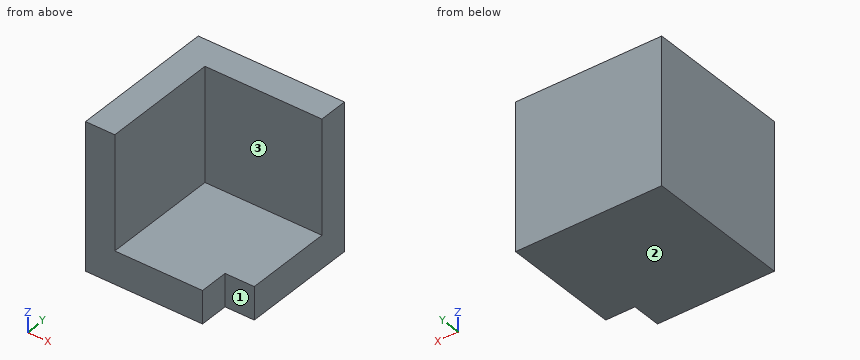
```python
from build123d import *

# Parameters (mm, degrees)
F0_W     = 63.5
F0_H     = 63.5
F1_DEPTH = 63.5
F2_W     = 50.8
F2_H     = 50.8
F3_DEPTH = 49.293023
F4_W     = 12.7
F4_H     = 12.7
F5_DEPTH = 25.4


with BuildPart() as f1:
    # F0 (on Front) → F1 (new body)
    with BuildSketch(Plane.XZ):
        with Locations((31.75, 31.75)):
            Rectangle(F0_W, F0_H)
    extrude(amount=F1_DEPTH)

    # F2 (on face) → F3 (cut)
    with BuildSketch(Plane.XY.offset(63.5)):
        with Locations((38.1, -38.1)):
            Rectangle(F2_W, F2_H)
    extrude(amount=-F3_DEPTH, mode=Mode.SUBTRACT)

    # F4 (on face) → F5 (cut)
    with BuildSketch(Plane.XY.offset(14.206977)):
        with Locations((57.15, -57.15)):
            Rectangle(F4_W, F4_H)
    extrude(amount=-F5_DEPTH, mode=Mode.SUBTRACT)


solid = f1.part
```
Here's how the part is built. I have some questions about the finished solid (model axes, mm). Face numbers are marked on the shaded views. A direction names the side the tool comes from. Round coordinates to 2 decimals unless told otherwise and drop trailing zeros. Order: outer loops, then holes, each group sorted by start corner. A loop starts at its lowest first (then second) coordinate and runs counter-clockwise, first axis right, second up. Notation, with made-up numbers: M 73.5,74.5 L 109.5,74.5 A36 ccw 109.5,108.5 Z; hole C 50.5,-35.75 d11. An arc over 180 degrees is marked long. Answer in a Markdown table with one row per item.
Item 1: Imagine slicing it at B-B, the plane x = 56.5. Write out the boundary of the cut face in (y, z).
A:
| item | result |
|---|---|
| outline | M -50.8,0 L 0,0 L 0,63.5 L -12.7,63.5 L -12.7,14.21 L -50.8,14.21 Z |
Item 2: If I drill on L1, parallel to X at y = -60, z = 20; L2, parallel to Y at x = 40, z = 40; L3, parallel to Z at x = 20, y = -32.5, over which ranges is the centre line in solid material (lowest first)? Write a range as from..to.
A:
| item | result |
|---|---|
| L1 | x = 0..12.7 |
| L2 | y = -12.7..0 |
| L3 | z = 0..14.21 |
Item 3: I'm going to push flat-ended pins straight in: pin 1 (10 mm diameter, centred on x = 41.5, z = 51.5, fed in from -Y); pin 2 (15 mm diameter, centred on x = 34, y = -47.5, fed in from +Z); pin 3 (10 mm diameter, centred on x = 56, z = 4.5, fed in from -Y). Where does each tip first touch, or does it pass through?
A:
| item | result |
|---|---|
| pin 1 | stops at y = -12.7 |
| pin 2 | stops at z = 14.21 |
| pin 3 | stops at y = -50.8 |
Item 4: For the marked faces 1, 2 and 3, which set-ups out of +Z, -Z, +X, -X, +Y, -Y let a thin tool reach every point of the face, with its end or its side?
A:
| item | result |
|---|---|
| face 1 | +Z, -Z, +X, -Y |
| face 2 | -Z, +X, -X, +Y, -Y |
| face 3 | +Z, +X, -Y |
Item 5: Imagine slicing it at A-A, the plane z = 39.5. Write out the boundary of the cut face in (x, y).
A:
| item | result |
|---|---|
| outline | M 0,-63.5 L 12.7,-63.5 L 12.7,-12.7 L 63.5,-12.7 L 63.5,0 L 0,0 Z |
